from build123d import *

# Parameters (mm, degrees)
F2_R     = 4.895
F3_DEPTH = 26.631
F4_R     = 0.5


with BuildPart() as f1:
    # F0 (on Front) → F1 (revolve)
    with BuildSketch(Plane.XZ):
        Polygon((-7.58, 0), (0, 0), (0, 26.63), (-7.58, 26.63), (-7.58, 23.38), (-7.23, 23.38), (-7.23, 22.28), (-7.58, 22.28), (-7.58, 4.35), (-7.23, 4.35), (-7.23, 3.25), (-7.58, 3.25), align=None)
    revolve(axis=Axis((0, 0, 13.315), (0, 0, 1)))

    # F2 (on face) → F3 (cut, through all)
    with BuildSketch(Plane.XY.offset(26.63)):
        Circle(F2_R)
    extrude(amount=-F3_DEPTH, mode=Mode.SUBTRACT)

    # F4
    f4_edges = [f1.edges().sort_by_distance(p)[0] for p in [
        (7.58, 0, 0),
        (7.58, 0, 26.63),
    ]]
    fillet(f4_edges, radius=F4_R)


solid = f1.part
Model file for the job. Use its own axes, mm. A direction names the side the tool comes from. Coordinates: 2 decimals unless noted, no trailing zeros. Write each loop counter-clockwise with the first axis right and the second up, starting at its lowest first coordinate (ties: lowest second). Pieces come first, ordered by that corner, then holes. Notation, with made-up numbers: (42, 63.5) -> (60, 63.5) arc R22 ccw to (60, 88.5) -> close; hole circle Ø5 at (-10, 20). An arc over 180 degrees is marked (long way). One line per item, written item: value. Start each with the question number.
1) Flat gauge pins, fed straight in: pin 1 Ø3 at (y, z) = (-5, 22.5) entering from +X; pin 2 Ø6 at (x, y) = (0, 0) entering from +Z; pin 3 Ø5 at (y, z) = (-6, 23.5) entering from -X. Where does each tip first touch, or does it go through?
2) Slice it at A-A on x = 0. Write the cut outline in (y, z) (3 decimals).
3) Probe probe 1 along Y at (x, z) = (0, 19.5) (3 decimals); probe 2 along Y at (x, z) = (1.5, 18.25); probe 3 along X at (y, z) = (4.5, 23). List the from-to ranges inside material, lowest first.
4) Which spindle directions (+Z, -Z, +X, -X, +Y, -Y) get a long thin tool onto all of the face, cutting with end or side? Do faces 1 (the face through (-6.68, 2.77, 22.82)), 2 (the face through (-7.23, -2.28, 24.74)). Say none if no direction does.
5) Pull direction X, two halves, no side cores. Call faces 3 (the face through (-2, 5, 26.63)), 4 (the face through (-7.23, -2.28, 13.19)), 5 (the face through (4.522, -1.875, 13.501)): +X half, -X half, draft (parallel to the pull), parting line (faces both ways), or undercut.
6) Slice it at C-C on z = 12. Write the cut outline in (x, y) (3 decimals).
Answers follow:
1. pin 1: x = 6.72
1. pin 2: through
1. pin 3: x = -6.72
2. outline: (-7.58, 0.5) arc R0.5 ccw to (-7.08, 0) -> (-4.895, 0) -> (-4.895, 26.63) -> (-7.08, 26.63) arc R0.5 ccw to (-7.58, 26.13) -> (-7.58, 23.38) -> (-7.23, 23.38) -> (-7.23, 22.28) -> (-7.58, 22.28) -> (-7.58, 4.35) -> (-7.23, 4.35) -> (-7.23, 3.25) -> (-7.58, 3.25) -> close; (4.895, 0) -> (7.08, 0) arc R0.5 ccw to (7.58, 0.5) -> (7.58, 3.25) -> (7.23, 3.25) -> (7.23, 4.35) -> (7.58, 4.35) -> (7.58, 22.28) -> (7.23, 22.28) -> (7.23, 23.38) -> (7.58, 23.38) -> (7.58, 26.13) arc R0.5 ccw to (7.08, 26.63) -> (4.895, 26.63) -> close
3. probe 1: -7.58 to -4.895, 4.895 to 7.58
3. probe 2: -7.43 to -4.66, 4.66 to 7.43
3. probe 3: -5.66 to -1.93, 1.93 to 5.66
4. face 1: none
4. face 2: +Z, -Z
5. face 3: draft
5. face 4: parting line
5. face 5: undercut
6. outline: circle Ø15.16 at (0, 0); hole circle Ø9.79 at (0, 0)
